The drawing under review shows one solid part. Ordinate dimensions are in mm from its lowest x, y, z. Give positions to 0.01 mm unless a question says otherwise; leave off trailing zeros. Write each loop counter-clockwise with the first axis right and the second up, starting at its lowest first coordinate (ties: lowest second). Pieces come first, ordered by that corner, then holes. Notation, with made-up numbers: (45, 86.25) -> (54, 86.25) arc R19 ccw to (54, 97.25) -> close; hole circle Ø2 at (65.25, 70). An arc over 180 degrees is marked (long way). Answer as a JSON object with one key per item and string values.
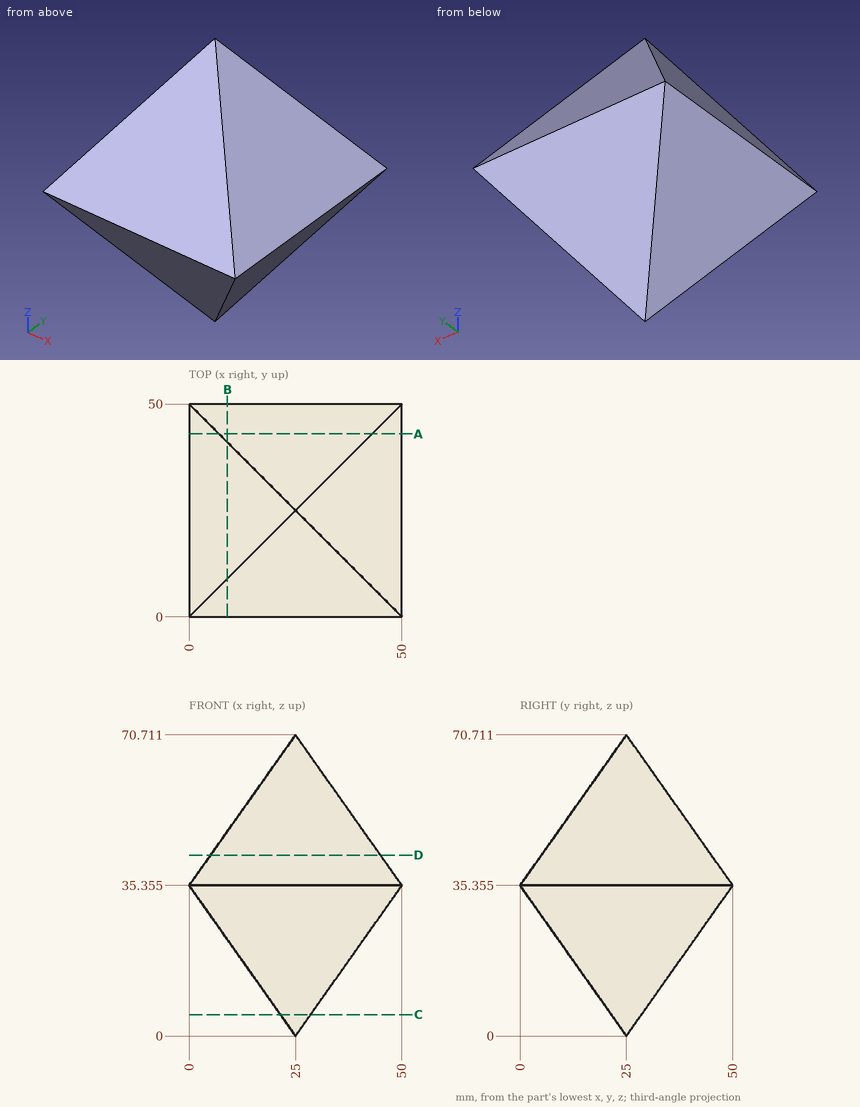
(1) We need section A-A, the plane y = 43. State the section outline as (x, z) points (1 decimal).
Here are the results:
{"outline": "(0, 35.4) -> (7, 25.5) -> (43, 25.5) -> (50, 35.4) -> (43, 45.3) -> (7, 45.3) -> close"}
(2) We need section B-B, the plane x = 9. State the section outline as (y, z) points (1 decimal).
Here are the results:
{"outline": "(0, 35.4) -> (9, 22.6) -> (41, 22.6) -> (50, 35.4) -> (41, 48.1) -> (9, 48.1) -> close"}
(3) We need section C-C, the plane z = 5. State the section outline as (x, y) points (1 decimal), then the cut area to 3 significant figures.
Here are the results:
{"outline": "(21.5, 21.5) -> (28.5, 21.5) -> (28.5, 28.5) -> (21.5, 28.5) -> close", "area": "50.0 mm²"}
(4) We need section D-D, the plane z = 42.5. State the section outline as (x, y) points, then the cut area to 3 significant figures.
Here are the results:
{"outline": "(5.05, 5.05) -> (44.95, 5.05) -> (44.95, 44.95) -> (5.05, 44.95) -> close", "area": "1,590 mm²"}
(5) For line 1 along Z through (x, y) = (3.5, 33) (1 decimal); line 2 along X through (y, z) = (8.5, 46.5); line 3 along X through (y, z) = (28, 11.5), list the stretches that pass through material, from the lowest coordinate up.
Here are the results:
{"line 1": "z = 30.4 to 40.3", "line 2": "x = 7.88 to 42.12", "line 3": "x = 16.87 to 33.13"}
(6) Clearance check with flat-ended pins moving along their axes: pin 1 (4 mm diameter, centred on x = 42.5, y = 15.5, fed in from +Z); pin 2 (6 mm diameter, centred on y = 36.5, z = 18.5, fed in from -X); pin 3 (1.5 mm diameter, centred on x = 15.5, y = 41.5, fed in from -Z) (1 decimal). State where each tip first meets the part, or that it passes through.
Here are the results:
{"pin 1": "stops at z = 48.79", "pin 2": "stops at x = 9.8", "pin 3": "stops at z = 22.3"}
